```python
from build123d import *

# Parameters (mm, degrees)
BOSS_CONFIGUP_DEPTH = 1.5875
FILLET1_R           = 1
FILLET2_R           = 1
FILLET3_R           = 0.5
FILLET4_R           = 0.25
FILLET5_R           = 2
FILLET7_R           = 1


with BuildPart() as part:
    # Sketch-ConfigUp → Boss-ConfigUp (new body, symmetric)
    with BuildSketch(Plane.XY):
        with BuildLine():
            Line((8.036884771, -1.932633536), (5.768256233, -2.958998264))
            ThreePointArc((5.768256233, -2.958998264), (5.166306437, -4.054514783), (3.946064636, -3.783387604))
            Line((3.946064636, -3.783387604), (0, -5.568651912))
            Line((0, -5.568651912), (0, -12.738236644))
            Line((0, -12.738236644), (16.372100646, -12.738236644))
            Line((16.372100646, -12.738236644), (16.372100646, -10.126726416))
            Line((16.372100646, -10.126726416), (13.32406834, -5.02866566))
            ThreePointArc((13.32406834, -5.02866566), (13.235492103, -3.587430718), (14.672142717, -3.442382733))
            Line((14.672142717, -3.442382733), (17.513873441, -0.098510164))
            ThreePointArc((17.513873441, -0.098510164), (17.370838202, 1.663460585), (15.608867453, 1.520425346))
            Line((15.608867453, 1.520425346), (13.685572067, -0.742721767))
            Line((13.685572067, -0.742721767), (11.665230115, 0.757902988))
            Line((11.665230115, 0.757902988), (9.20945182, 6.186040346))
            Line((9.20945182, 6.186040346), (8.77136122, 8.849335746))
            ThreePointArc((8.77136122, 8.849335746), (9.609835457, 9.662661067), (10.086138806, 10.729278263))
            ThreePointArc((10.086138806, 10.729278263), (9.52657217, 11.630324976), (8.625525457, 11.07075834))
            ThreePointArc((8.625525457, 11.07075834), (6.718309914, 9.886342294), (5.533893867, 11.793557837))
            ThreePointArc((5.533893867, 11.793557837), (4.974327231, 12.69460455), (4.073280517, 12.135037914))
            ThreePointArc((4.073280517, 12.135037914), (4.437375542, 9.835058641), (6.304511976, 8.443558952))
            Line((6.304511976, 8.443558952), (6.742602576, 5.780263553))
            Line((6.742602576, 5.780263553), (9.859076368, -1.108244196))
            ThreePointArc((9.859076368, -1.108244196), (9.257126572, -2.203760715), (8.036884771, -1.932633536))
        make_face()
        with BuildLine():
            Line((8.861274111, -3.754825133), (6.592645572, -4.781189861))
            ThreePointArc((6.592645572, -4.781189861), (5.372403771, -4.510062682), (4.770453975, -5.605579201))
            Line((4.770453975, -5.605579201), (4.770453975, -10.149803039))
            Line((4.770453975, -10.149803039), (6.154904632, -10.149803039))
            Line((6.154904632, -10.149803039), (11.419062352, -10.149803039))
            Line((11.419062352, -10.149803039), (13.32406834, -10.149803039))
            Line((13.32406834, -10.149803039), (11.419062352, -5.128381701))
            Line((11.419062352, -5.128381701), (11.419062352, -3.40973015))
            ThreePointArc((11.419062352, -3.40973015), (12.78717247, -3.341145376), (12.803247984, -1.971411553))
            Line((12.803247984, -1.971411553), (10.683465708, -2.930435793))
            ThreePointArc((10.683465708, -2.930435793), (9.463223907, -2.659308614), (8.861274111, -3.754825133))
        make_face(mode=Mode.SUBTRACT)
    extrude(amount=BOSS_CONFIGUP_DEPTH, both=True)

    # Fillet1
    fillet1_edges = [part.edges().sort_by_distance(p)[0] for p in [
        (0, -5.568651912, 0),
        (6.304511976, 8.443558952, 0),
        (8.77136122, 8.849335746, 0),
        (13.685572067, -0.742721767, 0),
    ]]
    fillet(fillet1_edges, radius=FILLET1_R)

    # Fillet2
    fillet2_edges = [part.edges().sort_by_distance(p)[0] for p in [
        (11.419062352, -3.40973015, 0),
    ]]
    fillet(fillet2_edges, radius=FILLET2_R)

    # Fillet3
    fillet3_edges = [part.edges().sort_by_distance(p)[0] for p in [
        (3.946064636, -3.783387604, 0),
        (5.768256233, -2.958998264, 0),
        (8.036884771, -1.932633536, 0),
        (14.672142717, -3.442382733, 0),
        (6.592645572, -4.781189861, 0),
        (10.683465708, -2.930435793, 0),
        (8.861274111, -3.754825133, 0),
    ]]
    fillet(fillet3_edges, radius=FILLET3_R)

    # Fillet4
    fillet4_edges = [part.edges().sort_by_distance(p)[0] for p in [
        (9.859076368, -1.108244196, 0),
        (12.803247984, -1.971411553, 0),
    ]]
    fillet(fillet4_edges, radius=FILLET4_R)

    # Fillet5
    fillet5_edges = [part.edges().sort_by_distance(p)[0] for p in [
        (6.742602576, 5.780263553, 0),
        (9.20945182, 6.186040346, 0),
        (11.665230115, 0.757902988, 0),
    ]]
    fillet(fillet5_edges, radius=FILLET5_R)

    # Fillet7
    fillet7_edges = [part.edges().sort_by_distance(p)[0] for p in [
        (4.770453975, -10.149803039, 0),
        (13.32406834, -10.149803039, 0),
    ]]
    fillet(fillet7_edges, radius=FILLET7_R)


solid = part.part
```
Read the model definition and answer for the solid it produces. Units are mm, in the model's axes. A direction names the side the tool comes from. Round coordinates to 2 decimals unless told otherwise and drop trailing zeros. Write each loop counter-clockwise with the first axis right and the second up, starting at its lowest first coordinate (ties: lowest second). Pieces come first, ordered by that corner, then holes. Notation, with made-up numbers: M 81,9 L 93,9 A22 ccw 93,38 Z; hole C 66,60 d8. An arc over 180 degrees is marked long. One line per item, written item: value.
Q1. For a pull along X with two mould halves and no side action, classify faces 6 (the flat face through (6.55, 6.96, 0.02)), 7 (the cylindrical face through (9.543, 11.626, 0.022)), 8 (the flat face through (9.02, 7.34, 0.02)), 9 (the cylindrical face through (5.18, -4.05, 0.02)) as +X half, -X half, draft (parallel to the pull), parting line (faces both ways), or undercut.
Data:
face 6: -X half
face 7: undercut
face 8: +X half
face 9: undercut
Q2. Which of the six approach directions +Z, -Z, +X, -X, +Y, -Y give full straight-line access (tool end or side, diameter ignored) to faces 1 (the cylindrical face through (9.741, 9.868, 0.022)), 2 (the flat face through (14.96, 0.757, 0.022)), 3 (the cylindrical face through (9.48, -2.65, 0.02)), 4 (the flat face through (8, -12.738, 0)), 5 (the cylindrical face through (0.155, -5.678, 0.022))?
Data:
face 1: +Z, -Z, +X
face 2: +Z, -Z, +Y
face 3: +Z, -Z
face 4: +Z, -Z, +X, -X, -Y
face 5: +Z, -Z, -X, +Y
Q3. Find section A-A on y = -7.75. Write down the section's boundary in (x, z), plus the area to 3 significant figures.
Data:
outline: M 0,-1.59 L 4.77,-1.59 L 4.77,1.59 L 0,1.59 Z; M 12.41,-1.59 L 14.95,-1.59 L 14.95,1.59 L 12.41,1.59 Z
area: 23.2 mm2
Q4. Flat-ended cylindrical pins translate along their axes: pin 1 Ø1.6 at (x, z) = (8, 0.5) entering from +Y; pin 2 Ø1.6 at (y, z) = (-7.5, -0.5) entering from +X. Find the tip coordinate at first contact, or state that the pin passes through.
Data:
pin 1: y = 11.4
pin 2: x = 15.28
Q5. Straight lines are drawn through the part: line 1 (Y direction, x = 5, z = 1.1); line 2 (Y direction, x = 6, z = 0.3); line 3 (X direction, y = -11.5, z = -0.85). For each, find the intervals that lie inside material, in ascending order. Write a range as [from, to].
Data:
line 1: [-12.74, -9.79], [-4.79, -4.11], [9.15, 12.69]
line 2: [-12.74, -10.15], [-4.44, -2.86], [8.51, 10.27]
line 3: [0, 16.37]
Q6. Find section B-B on x = 15.25. Write down the section's boundary in (y, z).
Data:
outline: M -12.74,-1.59 L -8.25,-1.59 L -8.25,1.59 L -12.74,1.59 Z; M -2.76,-1.59 L 1.1,-1.59 L 1.1,1.59 L -2.76,1.59 Z
Q7. Find section C-C on x = 2. Write down the section's boundary in (y, z), plus the area to 3 significant figures.
Data:
outline: M -12.74,-1.59 L -4.66,-1.59 L -4.66,1.59 L -12.74,1.59 Z
area: 25.6 mm2
